Could you check a few things on this model? Use its own coordinates, in mm. A direction names the side the tool comes from. Give positions to 0.01 mm unless a question says otherwise; leave off trailing zeros. Loops run counter-clockwise (first coordinate to the right, second up) from the corner with the lowest first, then second, coordinate; pieces in that order, holes last. Notation, with made-up numbers: M 80,33 L 107,33 A19 cw 107,46 Z; hole C 72.5,5 d5. An arc over 180 degrees is marked long. Use a Markdown table: item, result. Add a question column.
1) Suppose I cut it at A-A on y = 0. List the corners of the cut face in (x, z) for me.
2) Will these pins go through, and if not, where does the flat tip stop? pin 1 Ø0.8 at (x, z) = (25, -1) entering from -Y; pin 2 Ø3 at (x, y) = (24, 1) entering from -Z; pin 3 Ø2.5 at (x, y) = (25, 0) entering from +Z.
3) We'd pull the mould along Y, two halves only. Please class faces 1 (the cylindrical face through (25.042, 10.204, 0.641)), 2 (the flat face through (25, -3, 3)), 3 (the cylindrical face through (23.5, -0.07, 2.5)), 4 (the flat face through (25, 14.616, 1)): +Y half, -Y half, draft (parallel to the pull), parting line (faces both ways), or undercut.
4) Suppose I cut it at B-B on z = 1.25. List the corners of the cut face in (x, y) for me, and give its area (3 significant figures).
5) Suppose I cut it at D-D on z = 2.25. List the corners of the cut face in (x, y) for me.
6) Suppose I cut it at C-C on x = 25. List the corners of the cut face in (y, z) for me.
7) Which directions (+Z, -Z, +X, -X, +Y, -Y) give clear straight access to the entire face, cutting with the end or side of a thin tool? Please do faces 5 (the flat face through (25, 2, 0)), 6 (the flat face through (22, 6, 2)).
8) If I drill on line 1 along X through (y, z) = (0, 2.95); line 2 along Y through (x, z) = (25, 3.7); line 3 along Y through (x, z) = (24.05, 0.5), over which ranges is the centre line in solid material (lowest first)? Write a range as [from, to].
Autodesk Inventor part; units mm, degrees
ref_plane "YZ Plane" through (0, 0, 0) normal (1, 0, 0) x (0, 1, 0)
ref_plane "XZ Plane" through (0, 0, 0) normal (0, 1, 0) x (-1, 0, 0)
ref_plane "XY Plane" through (0, 0, 0) normal (0, 0, 1) x (1, 0, 0)
sketch "Sketch1" plane through (0, 0, 0) normal (0, 0, 1) x (1, 0, 0)
  circle A0 centre (25, 0) radius 1.5
  line L0 (30, 7.2167) -> (20.6, 7.2167)
  line L1 (30, 10.2167) -> (20.6, 10.2167)
  line L2 (22, -3) -> (28, -3)
  line L3 (28, -3) -> (22, -3)
  line L4 (22, -3) -> (22, 14.6155)
  line L5 (22, 14.6155) -> (28, 14.6155)
  line L6 (28, 14.6155) -> (28, -3)
  point P0 (0, 0)
extrude "Extrusion1" add sketch "Sketch1" along normal blind 5.08 and the other way blind 2.54
sketch "Sketch2" plane through (28, -3, 5.08) normal (1, 0, 0) x (0, 0, -1)
  line L0 (5.08, -1) -> (5.08, 7)
  circle A0 centre (4.6338, 11.7167) radius 1.5
  line L1 (5.08, 7) -> (7.62, 7)
  line L2 (7.62, 17.6155) -> (7.62, 0)
  line L3 (7.62, 7) -> (7.62, 0)
  line L4 (7.62, 0) -> (5.08, 0)
  line L5 (7.62, 0) -> (0, 0)
  line L6 (5.08, 0) -> (5.08, 7)
  point P0 (5.08, 3)
extrude "Extrusion2" cut sketch "Sketch2" against normal blind 7.62
properties part number "Base_encoder"
Answer block:
| question | item | result |
|---|---|---|
| 1 | outline | M 22,0 L 23.5,0 L 23.5,5.08 L 22,5.08 Z; M 26.5,0 L 28,0 L 28,5.08 L 26.5,5.08 Z |
| 2 | pin 1 | stops at y = 4 |
| 2 | pin 2 | stops at z = 0 |
| 2 | pin 3 | passes through |
| 3 | face 1 | undercut |
| 3 | face 2 | -Y half |
| 3 | face 3 | undercut |
| 3 | face 4 | +Y half |
| 4 | outline | M 22,-3 L 28,-3 L 28,7.45 L 22,7.45 Z; M 22,9.98 L 28,9.98 L 28,14.62 L 22,14.62 Z; hole C 25,0 d3 |
| 4 | area | 83.4 mm^2 |
| 5 | outline | M 22,-3 L 28,-3 L 28,14.62 L 22,14.62 Z; hole C 25,0 d3 |
| 6 | outline | M -3,0 L -1.5,0 L -1.5,5.08 L -3,5.08 Z; M 1.5,0 L 4,0 L 4,-2.54 L 14.62,-2.54 L 14.62,5.08 L 1.5,5.08 Z; hole C 8.72,0.45 d3 |
| 7 | face 5 | -Z, +X, -X, -Y |
| 7 | face 6 | +Z, -Z, -X, +Y, -Y |
| 8 | line 1 | x = [22, 23.5], [26.5, 28] |
| 8 | line 2 | y = [-3, -1.5], [1.5, 14.62] |
| 8 | line 3 | y = [-3, -1.16], [1.16, 7.22], [10.22, 14.62] |
